Work out the finished part from the listing and answer in its coordinate system (mm). A direction names the side the tool comes from. Coordinates: 2 decimals unless noted, no trailing zeros. Order: outer loops, then holes, each group sorted by start corner. A loop starts at its lowest first (then second) coordinate and runs counter-clockwise, first axis right, second up. Notation, with made-up numbers: M 7.5,6 L 46.5,6 A19 cw 46.5,42 Z; hole C 12.5,66.25 d11. An arc over 180 degrees is marked long. Write item = value, one per line. Start each with the question number.
Q1. Find section B-B on x = 33.5. Give the vertices of the cut face in (y, z), and give its area (3 significant figures).
Q2. A tool of negligible diameter and unlimited length cuts with its end or side. For faces 1 (the flat face through (40.821, 12, 3)), 2 (the flat face through (34, -9.73, 3)), 3 (the flat face through (27, 35.355, 3)), from which of +Z, -Z, +X, -X, +Y, -Y can it reach the whole face along a straight path? Write none if from no direction.
Q3. Straight lines are drawn through the part: line 1 along X through (y, z) = (28, 4.25); line 2 along Y through (x, z) = (34.25, 5.25); line 3 along Y through (x, z) = (27.5, 4.75). For each, find the intervals that lie inside material, in ascending order.
Q4. Find section A-A on z = 2. Give the vertices of the cut face in (x, y) (3 decimals), and give its area (3 significant figures).
Q5. Find section C-C on y = 2. Give the vertices of the cut face in (x, z), and give its area (3 significant figures).
Q6. Each of these flat-tipped pins is pushed along its axis until it touches: P1, Ø3, axis at x = 42.5, z = 3, coming from the -Y side; P2, Ø3, axis at y = 18, z = 3.5, coming from the -X side; P3, Ø1.9, axis at y = 21, z = 2.5, coming from the +X side; P4, Ø1, axis at x = 32, y = 17.5, coming from the -Z side. Where does it stop, or does it pass through?
Q7. Find section D-D on x = 41.5. Give the vertices of the cut face in (y, z), and give its area (3 significant figures).
```python
from build123d import *

# Parameters (mm, degrees)
F1_DEPTH = 6.35


with BuildPart() as f1:
    # F0 (on Top) → F1 (new body)
    with BuildSketch(Plane.XY):
        with BuildLine():
            Line((34.47086, -2.110446), (34.47086, -9.730446))
            Line((34.47086, -9.730446), (40.82086, -9.730446))
            Line((40.82086, -9.730446), (40.82086, 35.354554))
            Line((40.82086, 35.354554), (43.36086, 35.354554))
            Line((43.36086, 35.354554), (43.36086, 37.894554))
            Line((43.36086, 37.894554), (34.47086, 37.894554))
            Line((34.47086, 37.894554), (34.47086, 35.354554))
            Line((34.47086, 35.354554), (34.47086, 4.239554))
            ThreePointArc((34.47086, 4.239554), (36.715924, 3.309618), (37.64586, 1.064554))
            ThreePointArc((37.64586, 1.064554), (36.715924, -1.18051), (34.47086, -2.110446))
        make_face()
        with BuildLine():
            Line((28.12086, -9.730446), (34.47086, -9.730446))
            Line((34.47086, -9.730446), (34.47086, -2.110446))
            ThreePointArc((34.47086, -2.110446), (31.29586, 1.064554), (34.47086, 4.239554))
            Line((34.47086, 4.239554), (34.47086, 35.354554))
            Line((34.47086, 35.354554), (34.47086, 37.894554))
            Line((34.47086, 37.894554), (25.58086, 37.894554))
            Line((25.58086, 37.894554), (25.58086, 35.354554))
            Line((25.58086, 35.354554), (28.12086, 35.354554))
            Line((28.12086, 35.354554), (28.12086, -9.730446))
        make_face()
    extrude(amount=F1_DEPTH)


solid = f1.part
```
Findings below:
q1.outline = M -9.73,0 L -1.96,0 L -1.96,6.35 L -9.73,6.35 Z; M 4.09,0 L 37.89,0 L 37.89,6.35 L 4.09,6.35 Z
q1.area = 264 mm^2
q2.face_1 = +Z, -Z, +X, -Y
q2.face_2 = +Z, -Z, +X, -X, -Y
q2.face_3 = +Z, -Z, -X, -Y
q3.line_1 = 28.12 to 40.82
q3.line_2 = -9.73 to -2.1, 4.23 to 37.89
q3.line_3 = 35.35 to 37.89
q4.outline = M 25.581,35.355 L 28.121,35.355 L 28.121,-9.73 L 40.821,-9.73 L 40.821,35.355 L 43.361,35.355 L 43.361,37.895 L 25.581,37.895 Z; hole C 34.471,1.065 d6.35
q4.area = 586 mm^2
q5.outline = M 28.12,0 L 31.44,0 L 31.44,6.35 L 28.12,6.35 Z; M 37.5,0 L 40.82,0 L 40.82,6.35 L 37.5,6.35 Z
q5.area = 42.1 mm^2
q6.P1 = 35.35
q6.P2 = 28.12
q6.P3 = 40.82
q6.P4 = 0
q7.outline = M 35.35,0 L 37.89,0 L 37.89,6.35 L 35.35,6.35 Z
q7.area = 16.1 mm^2
